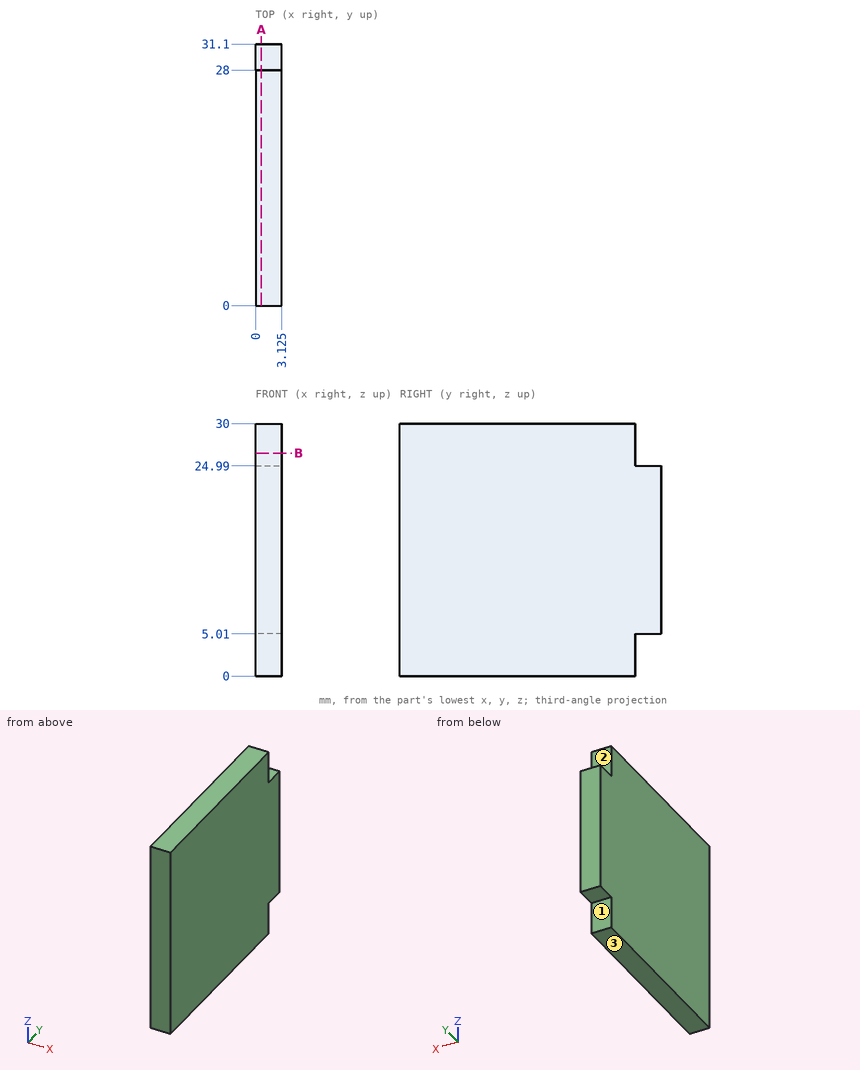
Check sheet for the drawn part. Datum: minimum x, y, z corner. Units: mm. A direction names the side the tool comes from. Round coordinates to 2 decimals unless told otherwise and drop trailing zeros. Loops run counter-clockwise (first coordinate to the right, second up) from the corner with the lowest first, then second, coordinate; pieces in that order, holes last. Notation, with made-up numbers: (87.25, 83.5) - (107.25, 83.5) arc R19 ccw to (107.25, 113.5) - close; hole circle Ø1 at (-22.75, 83). An arc over 180 degrees is marked (long way). Answer as a JSON object with one key per item and string values. Group by question number.
Q1. Set-up check for the marked faces 1, 2 and 3: record each of +Z, -Z, +X, -X, +Y, -Y from which the full face is reachable in a straight line by a thin tool's end or side.
Q2. Gauge pin test, flat end, axial feed: P1, Ø1.6, axis at x = 1, z = 28, coming from the +Y side. Record the tip position at first contact, or that the pin passes through.
Q3. Sectioned sample at A-A, the plane x = 0.7. Enter the section's corners in (y, z), plus the area to 3 significant figures.
Q4. Scan line: line 1 along Y through (x, z) = (0.25, 26). Record every from-to range of solid material in increasing order. Write a range as [from, to].
Q5. Sectioned sample at B-B, the plane z = 26.5. Enter the section's corners in (x, y) (3 decimals).
Solution:
{
 "1": {"face 1": "-Z, +X, -X, +Y", "face 2": "+Z, +X, -X, +Y", "face 3": "-Z, +X, -X, +Y, -Y"},
 "2": {"P1": "stops at y = 28"},
 "3": {"outline": "(0, 0) - (28, 0) - (28, 5.01) - (31.1, 5.01) - (31.1, 24.99) - (28, 24.99) - (28, 30) - (0, 30) - close", "area": "902 mm²"},
 "4": {"line 1": "y = [0, 28]"},
 "5": {"outline": "(0, 0) - (3.125, 0) - (3.125, 28) - (0, 28) - close"}
}
